```python
from build123d import *

# Parameters (mm, degrees)
F1_DEPTH = 25.4
F2_R     = 4.688974
F4_DEPTH = 25


with BuildPart() as f1:
    # F0 (on Front) → F1 (new body)
    with BuildSketch(Plane.XZ):
        Polygon((-46.851493, -26.17777), (-73.968977, -26.17777), (-53.295251, -47.388475), (47.656961, -47.388475), (62.423911, -26.17777), (13.290253, -26.17777), (0, -26.17777), (-21.61344, -26.17777), align=None)
        Polygon((-46.851493, -8.457433), (-46.851493, -26.17777), (-21.61344, -26.17777), (-21.61344, -17.049111), (-32.621529, -17.049111), (-32.621529, -8.457433), align=None)
    extrude(amount=F1_DEPTH)

    # F2 (on face) → F4 (join)
    with BuildSketch(Plane.XY.offset(-26.17777)):
        with Locations((13.558744, -12.484781)):
            Circle(F2_R)
    extrude(amount=F4_DEPTH)


solid = f1.part
```
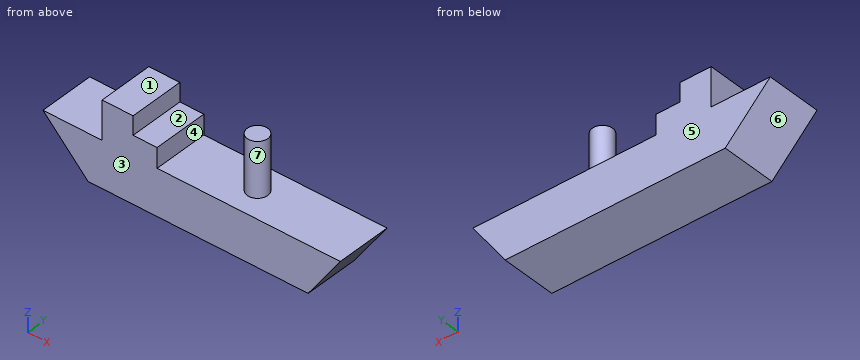
Read the model definition and answer for the solid it produces. Units are mm, in the model's axes. Face numbers are marked on the shaded views. A direction names the side the tool comes from. Give positions to 0.01 mm unless a question says otherwise; leave off trailing zeros. Write each loop counter-clockwise with the first axis right and the second up, starting at its lowest first coordinate (ties: lowest second). Pieces come first, ordered by that corner, then holes. Notation, with made-up numbers: (83, 77.25) -> (123, 77.25) arc R31 ccw to (123, 101.25) -> close; hole circle Ø9 at (49.5, -24.5). An arc over 180 degrees is marked (long way). Answer in a Markdown table with one row per item.
1) Section B-B on z = -19 is taken. Give the vertices of the cut face in (x, y), plus the area to 3 significant figures.
Results list:
| item | result |
|---|---|
| outline | (-46.85, -25.4) -> (-21.61, -25.4) -> (-21.61, 0) -> (-46.85, 0) -> close; circle Ø9.38 at (13.56, -12.48) |
| area | 710 mm^2 |
2) Each of these flat-tipped pins is pushed along its axis until it touches: pin 1 Ø4.5 at (y, z) = (-6.5, -22.5) entering from +X; pin 2 Ø2 at (y, z) = (-13.5, -12) entering from -X; pin 3 Ø5.5 at (x, y) = (-28.5, -6.5) entering from +Z. Where does it stop, or does it pass through?
Results list:
| item | result |
|---|---|
| pin 1 | x = 16.39 |
| pin 2 | x = -46.85 |
| pin 3 | z = -17.05 |
3) Section D-D on z = -43 is taken. Give the vertices of the cut face in (x, y).
Results list:
| item | result |
|---|---|
| outline | (-57.57, -25.4) -> (50.71, -25.4) -> (50.71, 0) -> (-57.57, 0) -> close |
4) Section A-A on y = -23 is taken. Give the vertices of the cut face in (x, z).
Results list:
| item | result |
|---|---|
| outline | (-73.97, -26.18) -> (-53.3, -47.39) -> (47.66, -47.39) -> (62.42, -26.18) -> (-21.61, -26.18) -> (-21.61, -17.05) -> (-32.62, -17.05) -> (-32.62, -8.46) -> (-46.85, -8.46) -> (-46.85, -26.18) -> close |
5) A tool of negligible diameter and unlimited length cuts with its end or side. For the marked faces 1, 2 and 3, from which of +Z, -Z, +X, -X, +Y, -Y can it reach the whole face along a straight path? Write none if from no direction.
Results list:
| item | result |
|---|---|
| face 1 | +Z, -X, +Y, -Y |
| face 2 | +Z, +Y, -Y |
| face 3 | +Z, -Z, +X, -X, -Y |
6) Determine the mould class of the marked faces 4, 5, 6 and 7 for opening direction X: released by +X, released by -X, zero draft, split by the parting line, or undercut.
Results list:
| item | result |
|---|---|
| face 4 | undercut |
| face 5 | zero draft |
| face 6 | released by -X |
| face 7 | undercut |
7) Section C-C on x = 1 is taken. Give the vertices of the cut face in (y, z).
Results list:
| item | result |
|---|---|
| outline | (-25.4, -47.39) -> (0, -47.39) -> (0, -26.18) -> (-25.4, -26.18) -> close |
8) Straight lines are drawn through the part: line 1 (Z direction, x = 25.5, y = -4.5); line 2 (X direction, y = -9.5, z = -22); line 3 (Z direction, x = -38, y = -3.5). For each, find the intervals that lie inside material, in ascending order. Write a range as [from, to].
Results list:
| item | result |
|---|---|
| line 1 | [-47.39, -26.18] |
| line 2 | [-46.85, -21.61], [9.94, 17.18] |
| line 3 | [-47.39, -8.46] |
